Geometry: see drawing. Coordinates: mm, zero at the bounding-box minimum. Round coordinates to 2 decimals unless told otherwise and drop trailing zeros. Loops run counter-clockwise (first coordinate to the right, second up) from the corner with the lowest first, then second, coordinate; pieces in that order, holes last. Notation, with made-up numbers: (-15.5, 14) - (40.5, 14) arc R24 ccw to (40.5, 34) - close; hole circle Ø9 at (59, 20). An arc over 180 degrees is marked (long way). Write item = value, one per line. Start each with the question number.
Item 1: Section A-A (x = 85). Return loops of the section in (y, z), plus the area to 3 significant figures.
Item 2: Section B-B (y = 1.05). Return loops of the section in (x, z).
Item 3: Section D-D (z = 38). Return loops of the section in (x, y).
Item 4: Section C-C (z = 75). Return loops of the section in (x, y).
Item 5: Line query: line 1 (X direction, y = 0.5, z = 84); line 2 (Z direction, x = 91, y = 1.05); line 3 (X direction, y = 1, z = 19). Output: solid intervals per line, ascending. Write a range as from..to.
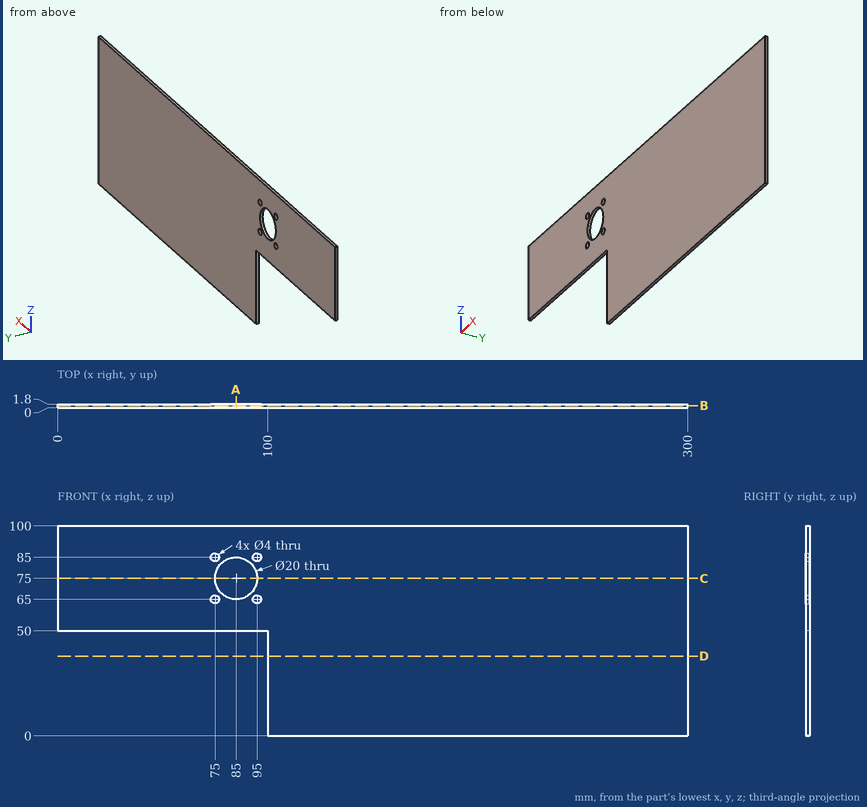
Taken from the geometry:
q1.outline = (0, 50) - (1.8, 50) - (1.8, 65) - (0, 65) - close; (0, 85) - (1.8, 85) - (1.8, 100) - (0, 100) - close
q1.area = 54.0 mm^2
q2.outline = (0, 50) - (100, 50) - (100, 0) - (300, 0) - (300, 100) - (0, 100) - close; hole circle Ø4 at (75, 65); hole circle Ø4 at (75, 85); hole circle Ø20 at (85, 75); hole circle Ø4 at (95, 65); hole circle Ø4 at (95, 85)
q3.outline = (100, 0) - (300, 0) - (300, 1.8) - (100, 1.8) - close
q4.outline = (0, 0) - (75, 0) - (75, 1.8) - (0, 1.8) - close; (95, 0) - (300, 0) - (300, 1.8) - (95, 1.8) - close
q5.line_1 = 0..73.27, 76.73..80.64, 89.36..93.27, 96.73..300
q5.line_2 = 50..67, 83..100
q5.line_3 = 100..300
